Can you work these out from the model? Positions are in its coordinate system, mm. A direction names the side the tool comes from. Round coordinates to 2 decimals unless told otherwise and drop trailing zeros. Write each loop counter-clockwise with the first axis right and the second up, starting at its lowest first coordinate (ties: lowest second). Pieces come first, ordered by that corner, then holes. Notation, with made-up numbers: (-14, 75) - (-1, 75) arc R15 ccw to (-1, 93) - close; hole circle Ø6 at (86, -27.75). An arc over 180 degrees is marked (long way). One line per item, written item: value. Start each with the question number.
(1) I'm going to push flat-ended pins straight in: pin 1 Ø3 at (y, z) = (56.99, -25.4) entering from +X; pin 2 Ø6 at (x, y) = (17, 36.5) entering from -Z. Where does each tip first touch, or does it pass through?
(2) On a 3-axis mill with a long thin cutter (end or side, diameter ignored), from which of +Z, -Z, +X, -X, +Y, -Y can I reach the whole of each face in a straight line? I mean faces 1 (the face through (6.35, 31, -22)), 2 (the face through (0, 31, -16)). Say none if no direction works.
(3) I want a section at B-B on y = 44.45. List the corners of the cut face in (x, z) for me, plus the area to 3 significant figures.
(4) I want a section at A-A on z = -20. List the corners of the cut face in (x, y) for me.
(5) Thinking about a two-plate mould opening in Z: for faces 3 (the face through (16, 31, 0)), 4 (the face through (16, 0, -13)), 5 (the face through (3.13, 59.13, -26.77)), which applies, +Z half, -Z half, draft (parallel to the pull), parting line (faces both ways), or undercut?
(6) I want a section at D-D on z = -25.4. List the corners of the cut face in (x, y) for me, plus the area to 3 significant figures.
(7) I want a section at C-C on x = 21. List the corners of the cut face in (y, z) for me, plus the area to 3 significant figures.
(8) If I drill on L1, parallel to Y at x = 1.5, z = -25.4; L2, parallel to X at y = 41, z = -23.5, over which ranges is the centre line in solid material (lowest first)? Write a range as from..to.
from build123d import *

# Parameters (mm, degrees)
BOSS_EXTRUDE1_DEPTH     = 63.5
SKETCH2_R               = 6.35
CUT_EXTRUDE1_DEPTH      = 79.25560529
CUT_EXTRUDE2_DEPTH      = 76.910329448
CUT_EXTRUDE2_DEPTH_BACK = 76.910329448
SKETCH5_R               = 3.302
SKETCH5_R_2             = 2.54


with BuildPart() as part:
    # Sketch1 → Boss-Extrude1 (new body)
    with BuildSketch(Plane(origin=(0, 0, 0), x_dir=(1, 0, 0), z_dir=(0, 1, 0))):
        Polygon((0, 0), (0, 33.02), (6.35, 33.02), (6.35, 17.78), (25.294420667, 17.78), (25.294420667, 33.02), (31.644420667, 33.02), (31.644420667, 0), align=None)
    extrude(amount=BOSS_EXTRUDE1_DEPTH)

    # Sketch2 → Cut-Extrude1 (cut, through all)
    with BuildSketch(Plane.XY):
        with Locations((15.822210333, 44.45)):
            Circle(SKETCH2_R)
        with Locations((15.822210333, 19.05)):
            Circle(SKETCH2_R)
    extrude(amount=-CUT_EXTRUDE1_DEPTH, mode=Mode.SUBTRACT)

    # Sketch5 → Cut-Extrude2 (cut, two sides: drawn at the far end of the back side and taken through both)
    with BuildSketch(Plane(origin=(6.35, 0, 0), x_dir=(0, 0, -1), z_dir=(1, 0, 0)).offset(-CUT_EXTRUDE2_DEPTH_BACK)):
        with Locations((25.4, 31.75)):
            Circle(SKETCH5_R)
        with Locations((25.4, 56.989992478)):
            Circle(SKETCH5_R_2)
    extrude(amount=CUT_EXTRUDE2_DEPTH + CUT_EXTRUDE2_DEPTH_BACK, mode=Mode.SUBTRACT)


solid = part.part
Established:
1. pin 1: through
1. pin 2: z = -17.78
2. face 1: -Z, +Y, -Y
2. face 2: +Z, -Z, -X, +Y, -Y
3. outline: (0, -33.02) - (6.35, -33.02) - (6.35, -17.78) - (9.47, -17.78) - (9.47, 0) - (0, 0) - close; (22.17, -17.78) - (25.29, -17.78) - (25.29, -33.02) - (31.64, -33.02) - (31.64, 0) - (22.17, 0) - close
3. area: 530 mm2
4. outline: (0, 0) - (6.35, 0) - (6.35, 63.5) - (0, 63.5) - close; (25.29, 0) - (31.64, 0) - (31.64, 63.5) - (25.29, 63.5) - close
5. face 3: +Z half
5. face 4: draft
5. face 5: undercut
6. outline: (0, 0) - (6.35, 0) - (6.35, 28.45) - (0, 28.45) - close; (0, 35.05) - (6.35, 35.05) - (6.35, 54.45) - (0, 54.45) - close; (0, 59.53) - (6.35, 59.53) - (6.35, 63.5) - (0, 63.5) - close; (25.29, 0) - (31.64, 0) - (31.64, 28.45) - (25.29, 28.45) - close; (25.29, 35.05) - (31.64, 35.05) - (31.64, 54.45) - (25.29, 54.45) - close; (25.29, 59.53) - (31.64, 59.53) - (31.64, 63.5) - (25.29, 63.5) - close
6. area: 658 mm2
7. outline: (0, -17.78) - (15.37, -17.78) - (15.37, 0) - (0, 0) - close; (22.73, -17.78) - (40.77, -17.78) - (40.77, 0) - (22.73, 0) - close; (48.13, -17.78) - (63.5, -17.78) - (63.5, 0) - (48.13, 0) - close
7. area: 868 mm2
8. L1: 0..28.45, 35.05..54.45, 59.53..63.5
8. L2: 0..6.35, 25.29..31.64
